Design review of the part built by this model. Coordinates are the model's own, in mm. Face numbers are marked on the shaded views. A direction names the side the tool comes from. Coordinates: 2 decimals unless noted, no trailing zeros. Order: outer loops, then holes, each group sorted by start corner. A loop starts at its lowest first (then second) coordinate and runs counter-clockwise, first axis right, second up. Notation, with made-up numbers: M 58.25,52 L 116.25,52 A16 ccw 116.25,83 Z; hole C -34,-27 d2. An arc over 180 degrees is marked long. Answer as a JSON object with one key per item and string values.
from build123d import *

# Parameters (mm, degrees)
PAD_DEPTH       = 10
SKETCH001_R     = 19
POCKET_DEPTH    = 10.001
SKETCH002_R     = 6
POCKET001_DEPTH = 10.001
FILLET_R        = 3
SKETCH003_R     = 3
POCKET002_DEPTH = 15
SKETCH004_R     = 3
POCKET003_DEPTH = 10.001


with BuildPart() as part:
    # Sketch → Pad (new body)
    with BuildSketch(Plane.XY):
        Polygon((0, 0), (0, 120), (29, 120), (29, 88.5), (48, 88.5), (48, 31.5), (29, 31.5), (29, 0), align=None)
    extrude(amount=-PAD_DEPTH)

    # Sketch001 → Pocket (cut, through all)
    with BuildSketch(Plane.XY):
        with Locations((19.5, 60)):
            Circle(SKETCH001_R)
    extrude(amount=-POCKET_DEPTH, mode=Mode.SUBTRACT)

    # Sketch002 → Pocket001 (cut, through all)
    with BuildSketch(Plane.XY):
        with Locations((12.5, 99.5)):
            Circle(SKETCH002_R)
        with Locations((12.5, 20.5)):
            Circle(SKETCH002_R)
    extrude(amount=-POCKET001_DEPTH, mode=Mode.SUBTRACT)

    # Fillet
    fillet_edges = [part.edges().sort_by_distance(p)[0] for p in [
        (29, 31.5, -5),
        (29, 88.5, -5),
        (48, 31.5, -5),
        (48, 88.5, -5),
    ]]
    fillet(fillet_edges, radius=FILLET_R)

    # Sketch003 → Pocket002 (cut)
    with BuildSketch(Plane(origin=(0, 0, 0), x_dir=(0, -1, 0), z_dir=(-1, 0, 0))):
        with Locations((-111, -5.5)):
            Circle(SKETCH003_R)
        with Locations((-87, -5.5)):
            Circle(SKETCH003_R)
        with Locations((-33, -5.5)):
            Circle(SKETCH003_R)
        with Locations((-9, -5.5)):
            Circle(SKETCH003_R)
    extrude(amount=-POCKET002_DEPTH, mode=Mode.SUBTRACT)

    # Sketch004 → Pocket003 (cut, through all)
    with BuildSketch(Plane.XY):
        with Locations((43.5, 84)):
            Circle(SKETCH004_R)
        with Locations((43.5, 36)):
            Circle(SKETCH004_R)
    extrude(amount=-POCKET003_DEPTH, mode=Mode.SUBTRACT)


solid = part.part
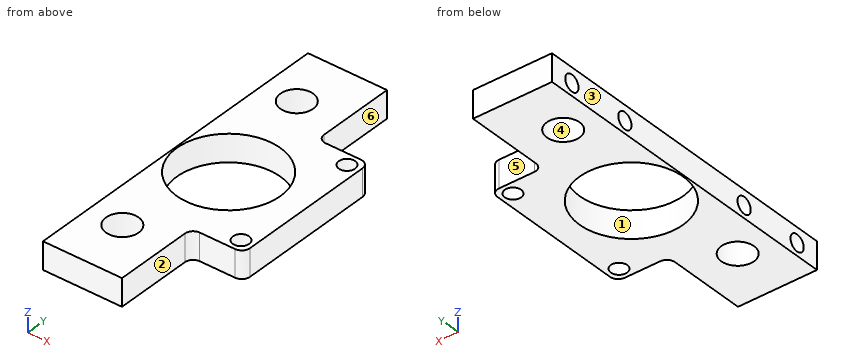
1) Add section D-D (y = 9). State the section outline as (x, z) points, and give its area (3 significant figures).
Taken from the geometry:
{"outline": "M 0,-10 L 29,-10 L 29,0 L 0,0 L 0,-2.5 L 15,-2.5 L 15,-8.5 L 0,-8.5 Z", "area": "200 mm2"}
2) Mouldability with a two-part tool opening along X and no side actions: class the marked faces 3, 4, 5 and 6 as released by +X, released by -X, zero draft, split by the parting line, or undercut.
Taken from the geometry:
{"face 3": "released by -X", "face 4": "undercut", "face 5": "zero draft", "face 6": "released by +X"}
3) Add section B-B (x = 43.5). State the section outline as (y, z) points.
Taken from the geometry:
{"outline": "M 31.5,-10 L 33,-10 L 33,0 L 31.5,0 Z; M 39,-10 L 81,-10 L 81,0 L 39,0 Z; M 87,-10 L 88.5,-10 L 88.5,0 L 87,0 Z"}
4) To check wall thickness, follow L1, parallel to X at y = 60.5, z = -4.75; L2, parallel to Y at x = 42.5, z = -1.25; L3, parallel to Z at x = 5, y = 111. State the ranges of each line that lie inside material, in increasing order.
Taken from the geometry:
{"L1": "x = 0 to 0.51, 38.49 to 48", "L2": "y = 31.5 to 33.17, 38.83 to 81.17, 86.83 to 88.5", "L3": "z = -10 to -8.5, -2.5 to 0"}
5) Insertion check: pin 1 Ø2 at (y, z) = (75, -6) entering from -X; pin 2 Ø5 at (y, z) = (14, -4.5) entering from +X; pin 3 Ø3 at (x, z) = (40.5, -7.5) entering from +Y; pin 4 Ø3 at (y, z) = (9, -6.5) entering from -X. Each pin has a flat end and moves straight along its axis. Give the tip position at first contact, or say it passes through.
Taken from the geometry:
{"pin 1": "stops at x = 0", "pin 2": "stops at x = 29", "pin 3": "stops at y = 88.5", "pin 4": "stops at x = 15"}
6) Add section A-A (y = 60). State the section outline as (x, z) points.
Taken from the geometry:
{"outline": "M 0,-10 L 0.5,-10 L 0.5,0 L 0,0 Z; M 38.5,-10 L 48,-10 L 48,0 L 38.5,0 Z"}
7) Tool access review of the marked faces 1 and 2: name each direction out of +Z, -Z, +X, -X, +Y, -Y from which nothing blocks a thin tool from reaching the whole face with its end or side.
Taken from the geometry:
{"face 1": "+Z, -Z", "face 2": "+Z, -Z, +X, -Y"}
8) Add section C-C (x = 20.5). State the section outline as (y, z) points.
Taken from the geometry:
{"outline": "M 0,-10 L 41.03,-10 L 41.03,0 L 0,0 Z; M 78.97,-10 L 120,-10 L 120,0 L 78.97,0 Z"}
